from build123d import *

# Parameters (mm, degrees)
SKETCH1_W                 = 10.15
SKETCH1_H                 = 18
SKETCH1_W_2               = 69.7
BOSS_EXTRUDE1_DEPTH       = 3
SKETCH1_3_W               = 69.7
SKETCH1_3_H               = 18
BOSS_EXTRUDE2_DEPTH       = 8
M3_CLEARANCE_HOLE1_D      = 3.6
M3_CLEARANCE_HOLE1_DEPTH  = 10
M3_CLEARANCE_HOLE1_TIP    = 1.081549114
SKETCH6_W                 = 69.7
SKETCH6_H                 = 37
BOSS_EXTRUDE3_DEPTH       = 5
BOSS_EXTRUDE4_DEPTH       = 3
F_3_0MM_DOWEL_HOLE1_D     = 3.5
F_3_0MM_DOWEL_HOLE1_DEPTH = 6
F_3_0MM_DOWEL_HOLE1_TIP   = 1.051506083
SKETCH12_W                = 50
SKETCH12_H                = 30
CUT_EXTRUDE1_DEPTH        = 65.845971347
CUT_EXTRUDE2_DEPTH        = 93.498770262
SKETCH15_W                = 69.7
SKETCH15_H                = 3
CUT_EXTRUDE3_DEPTH        = 2
CUT_EXTRUDE4_DEPTH        = 0.4


with BuildPart() as part:
    # Sketch1 → Boss-Extrude1 (new body)
    with BuildSketch(Plane(origin=(0, 0, 0), x_dir=(1, 0, 0), z_dir=(0, 1, 0))):
        with Locations((-39.925, 0)):
            Rectangle(SKETCH1_W, SKETCH1_H)
        Rectangle(SKETCH1_W_2, SKETCH1_H)
        with Locations((39.925, 0)):
            Rectangle(SKETCH1_W, SKETCH1_H)
    extrude(amount=BOSS_EXTRUDE1_DEPTH)

    # Sketch1_3 → Boss-Extrude2 (add)
    with BuildSketch(Plane(origin=(0, 0, 0), x_dir=(1, 0, 0), z_dir=(0, 1, 0))):
        Rectangle(SKETCH1_3_W, SKETCH1_3_H)
    extrude(amount=BOSS_EXTRUDE2_DEPTH)

    # M3 Clearance Hole1
    with Locations(Plane(origin=(0, 3, 0), x_dir=(1, 0, 0), z_dir=(0, 1, 0))):
        with Locations((-40, 5), (-40, -5), (40, -5), (40, 5)):
            Hole(M3_CLEARANCE_HOLE1_D / 2, depth=M3_CLEARANCE_HOLE1_DEPTH)
            with Locations((0, 0, -(M3_CLEARANCE_HOLE1_DEPTH + M3_CLEARANCE_HOLE1_TIP / 2))):  # 118° drill point
                Cone(0, M3_CLEARANCE_HOLE1_D / 2, M3_CLEARANCE_HOLE1_TIP, mode=Mode.SUBTRACT)

    # Sketch6 → Boss-Extrude3 (add)
    with BuildSketch(Plane.XZ):
        with Locations((0, -27.5)):
            Rectangle(SKETCH6_W, SKETCH6_H)
    extrude(amount=-BOSS_EXTRUDE3_DEPTH)

    # Sketch9 → Boss-Extrude4 (add)
    with BuildSketch(Plane.XZ):
        with BuildLine():
            ThreePointArc((34.85, -36.763103338), (33.735397376, -36.195556108), (32.5, -36))
            Line((32.5, -36), (32.5, -40))
            Line((32.5, -40), (28.5, -40))
            ThreePointArc((28.5, -40), (30.683409788, -43.563705936), (34.85, -43.236896662))
            Line((34.85, -43.236896662), (34.85, -36.763103338))
        make_face()
        with BuildLine():
            Line((32.5, -40), (32.5, -36))
            ThreePointArc((32.5, -36), (29.671572875, -37.171572875), (28.5, -40))
            Line((28.5, -40), (32.5, -40))
        make_face()
        with BuildLine():
            Line((-32.5, -40), (-32.5, -36))
            ThreePointArc((-32.5, -36), (-33.735397376, -36.195556108), (-34.85, -36.763103338))
            Line((-34.85, -36.763103338), (-34.85, -43.236896662))
            ThreePointArc((-34.85, -43.236896662), (-30.683409788, -43.563705936), (-28.5, -40))
            Line((-28.5, -40), (-32.5, -40))
        make_face()
        with BuildLine():
            ThreePointArc((-28.5, -40), (-29.671572875, -37.171572875), (-32.5, -36))
            Line((-32.5, -36), (-32.5, -40))
            Line((-32.5, -40), (-28.5, -40))
        make_face()
        with BuildLine():
            ThreePointArc((-32.5, 1), (-29.671572875, 2.171572875), (-28.5, 5))
            Line((-28.5, 5), (-32.5, 5))
            Line((-32.5, 5), (-32.5, 1))
        make_face()
        with BuildLine():
            Line((-32.5, 5), (-28.5, 5))
            ThreePointArc((-28.5, 5), (-29.671572856, 7.828427105), (-32.499999945, 9))
            ThreePointArc((-32.499999945, 9), (-36.5, 5.000000027), (-32.5, 1))
            Line((-32.5, 1), (-32.5, 5))
        make_face()
        with BuildLine():
            ThreePointArc((-32.5, 1), (-29.671572875, 2.171572875), (-28.5, 5))
            Line((-28.5, 5), (-32.5, 5))
            Line((-32.5, 5), (-32.5, 1))
        make_face()
        with BuildLine():
            Line((-32.5, 5), (-28.5, 5))
            ThreePointArc((-28.5, 5), (-29.671572856, 7.828427105), (-32.499999945, 9))
            ThreePointArc((-32.499999945, 9), (-36.5, 5.000000027), (-32.5, 1))
            Line((-32.5, 1), (-32.5, 5))
        make_face()
        with BuildLine():
            ThreePointArc((32.5, 9), (29.671572875, 7.828427125), (28.5, 5))
            Line((28.5, 5), (32.5, 5))
            Line((32.5, 5), (32.5, 1))
            ThreePointArc((32.5, 1), (35.328427125, 2.171572875), (36.5, 5))
            ThreePointArc((36.5, 5), (35.328427125, 7.828427125), (32.5, 9))
        make_face()
        with BuildLine():
            Line((32.5, 5), (28.5, 5))
            ThreePointArc((28.5, 5), (29.671572875, 2.171572875), (32.5, 1))
            Line((32.5, 1), (32.5, 5))
        make_face()
        with BuildLine():
            ThreePointArc((32.5, 9), (29.671572875, 7.828427125), (28.5, 5))
            Line((28.5, 5), (32.5, 5))
            Line((32.5, 5), (32.5, 1))
            ThreePointArc((32.5, 1), (35.328427125, 2.171572875), (36.5, 5))
            ThreePointArc((36.5, 5), (35.328427125, 7.828427125), (32.5, 9))
        make_face()
        with BuildLine():
            Line((32.5, 5), (28.5, 5))
            ThreePointArc((28.5, 5), (29.671572875, 2.171572875), (32.5, 1))
            Line((32.5, 1), (32.5, 5))
        make_face()
    extrude(amount=BOSS_EXTRUDE4_DEPTH)

    # 3.0mm Dowel Hole1
    with Locations(Plane(origin=(0, -3, 0), x_dir=(-1, 0, 0), z_dir=(0, -1, 0))):
        with Locations((-32.5, -5), (32.5, -5), (32.5, 40), (-32.5, 40)):
            Hole(F_3_0MM_DOWEL_HOLE1_D / 2, depth=F_3_0MM_DOWEL_HOLE1_DEPTH)
            with Locations((0, 0, -(F_3_0MM_DOWEL_HOLE1_DEPTH + F_3_0MM_DOWEL_HOLE1_TIP / 2))):  # 118° drill point
                Cone(0, F_3_0MM_DOWEL_HOLE1_D / 2, F_3_0MM_DOWEL_HOLE1_TIP, mode=Mode.SUBTRACT)

    # Sketch12 → Cut-Extrude1 (cut, through all)
    with BuildSketch(Plane.XZ):
        with Locations((0, -21)):
            Rectangle(SKETCH12_W, SKETCH12_H)
    extrude(amount=-CUT_EXTRUDE1_DEPTH, mode=Mode.SUBTRACT)

    # Sketch14 → Cut-Extrude2 (cut, through all)
    with BuildSketch(Plane.ZY.offset(34.85)):
        Polygon((9, 3), (9, 8), (-9, 8), (-9, 5), (-46, 5), (-46, 3), (-9, 3), align=None)
    extrude(amount=-CUT_EXTRUDE2_DEPTH, mode=Mode.SUBTRACT)

    # Sketch15 → Cut-Extrude3 (cut)
    with BuildSketch(Plane(origin=(0, 0, -46), x_dir=(-1, 0, 0), z_dir=(0, 0, -1))):
        with Locations((0, 1.5)):
            Rectangle(SKETCH15_W, SKETCH15_H)
    extrude(amount=-CUT_EXTRUDE3_DEPTH, mode=Mode.SUBTRACT)

    # Sketch16 → Cut-Extrude4 (cut)
    with BuildSketch(Plane(origin=(34.85, 0, 0), x_dir=(0, 0, -1), z_dir=(1, 0, 0))):
        Polygon((43.236896662, 0), (44, 0), (44, 3), (9, 3), (9, 0), (36.763103338, 0), (36.763103338, -3), (43.236896662, -3), align=None)
        Polygon((44, -5.236372104), (44, 0), (43.236896662, 0), (43.236896662, -3), (36.763103338, -3), (36.763103338, 0), (9, 0), (9, -5.236372104), align=None)
    cut_extrude4 = extrude(amount=-CUT_EXTRUDE4_DEPTH, mode=Mode.SUBTRACT)

    # Mirror1: Cut-Extrude4 across plane
    add(cut_extrude4.mirror(Plane(origin=(0, 0, 0), x_dir=(0, 0, 1), z_dir=(1, 0, 0))), mode=Mode.SUBTRACT)


solid = part.part
The listing builds one solid part. Answer for the finished solid, in the listing's coordinates (mm). A direction names the side the tool comes from. Give positions to 0.01 mm unless a question says otherwise; leave off trailing zeros. Write each loop counter-clockwise with the first axis right and the second up, starting at its lowest first coordinate (ties: lowest second). Pieces come first, ordered by that corner, then holes. Notation, with made-up numbers: (11.5, -31) -> (68.5, -31) arc R30 cw to (68.5, 6) -> close; hole circle Ø3 at (-13, 27.5). An arc over 180 degrees is marked (long way). Use a Markdown table: item, result.
(1) Find the intervals of material crossed by probe 1 along Z at (x, y) = (32.5, -1.5); probe 2 along X at (y, z) = (-1.75, -40); probe 3 along Z at (x, y) = (-40, 0.85), in increasing order. Write a range as from..to.
Return value:
| item | result |
|---|---|
| probe 1 | -44..-41.75, -38.25..-36, 1..3.25, 6.75..9 |
| probe 2 | -34.45..-34.25, -30.75..-28.5, 28.5..30.75, 34.25..34.45 |
| probe 3 | -9..-6.8, -3.2..3.2, 6.8..9 |
(2) Section D-D, the plane x = -4.5 is taken. Determine the outline of the cut face in (y, z), then the cut area to 3 significant figures.
Return value:
| item | result |
|---|---|
| outline | (0, -44) -> (3, -44) -> (3, -36) -> (0, -36) -> close; (0, -6) -> (3, -6) -> (3, 9) -> (0, 9) -> close |
| area | 69.0 mm2 |
(3) Flat-ended cylindrical pins translate along their axes: P1, Ø2, axis at x = 22.5, z = -3, coming from the -Y side; P2, Ø2.5, axis at x = -40, y = 1.5, coming from the -Z side; P3, Ø1.5, axis at y = 1, z = -27.5, coming from the -X side; P4, Ø5.5, axis at x = -32.5, z = 5, coming from the -Y side. Find the tip coordinate at first contact, or state that the pin passes through.
Return value:
| item | result |
|---|---|
| P1 | y = 0 |
| P2 | z = -9 |
| P3 | x = -34.45 |
| P4 | y = -3 |
(4) Section B-B, the plane x = -40 is taken. Determine the outline of the cut face in (y, z), then the cut area to 3 significant figures.
Return value:
| item | result |
|---|---|
| outline | (0, -9) -> (3, -9) -> (3, -6.8) -> (0, -6.8) -> close; (0, -3.2) -> (3, -3.2) -> (3, 3.2) -> (0, 3.2) -> close; (0, 6.8) -> (3, 6.8) -> (3, 9) -> (0, 9) -> close |
| area | 32.4 mm2 |
(5) Determine the mould class of faces 4 (the flat face through (-45, 1, 0)), 5 (the cylindrical face through (-34.25, 0.04, 4.92)), 6 (the cylindrical face through (39.169, 1.479, -3.403)), 7 (the flat face through (-40, 1, -9)) for opening direction Z: released by +Z, released by -Z, zero draft, split by the parting line, or undercut.
Return value:
| item | result |
|---|---|
| face 4 | zero draft |
| face 5 | undercut |
| face 6 | undercut |
| face 7 | released by -Z |
(6) For faces 1 (the flat face through (34.45, 1, -30)), 2 (the flat face through (-1, 0, -5)), 3 (the flat face through (0, 1, -6)), determine the directions among +Z, -Z, +X, -X, +Y, -Y from which every point of the face is accessible in a straight line to the end or side of a thin tool.
Return value:
| item | result |
|---|---|
| face 1 | -Z, +X, +Y, -Y |
| face 2 | -Y |
| face 3 | +Y, -Y |
(7) Section A-A, the plane y = -2 is taken. Determine the outline of the cut face in (x, z).
Return value:
| item | result |
|---|---|
| outline | circle Ø8 at (-32.5, 5); (-34.45, -43.49) arc R4 ccw (long way) to (-34.45, -36.51) -> close; circle Ø8 at (32.5, 5); (34.45, -43.49) -> (34.45, -36.51) arc R4 ccw (long way) to start; hole circle Ø3.5 at (-32.5, -40); hole circle Ø3.5 at (-32.5, 5); hole circle Ø3.5 at (32.5, -40); hole circle Ø3.5 at (32.5, 5) |
(8) Section C-C, the plane z = -33 is taken. Determine the outline of the cut face in (x, y), then the cut area to 3 significant figures.
Return value:
| item | result |
|---|---|
| outline | (-34.45, 0) -> (-25, 0) -> (-25, 3) -> (-34.45, 3) -> close; (25, 0) -> (34.45, 0) -> (34.45, 3) -> (25, 3) -> close |
| area | 56.7 mm2 |
